The listing builds one solid part. Answer for the finished solid, in the listing's coordinates (mm). A direction names the side the tool comes from. Coordinates: 2 decimals unless noted, no trailing zeros. Loops run counter-clockwise (first coordinate to the right, second up) from the corner with the lowest first, then second, coordinate; pieces in that order, holes last. Notation, with made-up numbers: (59, 9.5) - (64, 9.5) arc R9 ccw to (64, 17.5) - close; hole circle Ø5 at (73, 78). An arc over 180 degrees is marked (long way). Use one line per item in the form item = value. Start each with the question number.
```python
from build123d import *

# Parameters (mm, degrees)
ESQUISSE1_R                  = 13
BASE_EXTRUSION_DEPTH         = 5
ESQUISSE2_R                  = 5
BOSS_EXTRU_1_DEPTH           = 1.1
ESQUISSE3_R                  = 4
BOSS_EXTRU_2_DEPTH           = 16
ESQUISSE4_R                  = 3.5
BOSS_EXTRU_3_DEPTH           = 15
ESQUISSE5_R                  = 2
ENL_V_MAT_EXTRU_1_DEPTH      = 6
R_P_TITION_CIRCULAIRE1_COUNT = 3
ESQUISSE6_W                  = 3.116395494
ESQUISSE6_H                  = 0.94
CHANFREIN1_SIZE              = 0.5
ENL_V_MAT_EXTRU_2_DEPTH      = 10
ESQUISSE9_R                  = 6
ENL_V_MAT_EXTRU_3_DEPTH      = 1


with BuildPart() as part:
    # Esquisse1 → Base-Extrusion (new body)
    with BuildSketch(Plane.XY):
        Circle(ESQUISSE1_R)
    extrude(amount=BASE_EXTRUSION_DEPTH)

    # Esquisse2 → Boss.-Extru.1 (add)
    with BuildSketch(Plane.XY.offset(5)):
        Circle(ESQUISSE2_R)
    extrude(amount=BOSS_EXTRU_1_DEPTH)

    # Esquisse3 → Boss.-Extru.2 (add)
    with BuildSketch(Plane.XY.offset(6.1)):
        Circle(ESQUISSE3_R)
    extrude(amount=BOSS_EXTRU_2_DEPTH)

    # Esquisse4 → Boss.-Extru.3 (add)
    with BuildSketch(Plane.XY.offset(22.1)):
        Circle(ESQUISSE4_R)
    extrude(amount=BOSS_EXTRU_3_DEPTH)

    # Esquisse5 → Enlèv. mat.-Extru.1 (cut, through all)
    with BuildSketch(Plane.XY.offset(5)):
        with Locations((0, 9.75)):
            Circle(ESQUISSE5_R)
    enl_v_mat_extru_1 = extrude(amount=-ENL_V_MAT_EXTRU_1_DEPTH, mode=Mode.SUBTRACT)

    # Répétition circulaire1: Enlèv. mat.-Extru.1 ×3 about axis
    r_p_tition_circulaire1_axis = Axis((0, 0, 0), (0, 0, -1))
    for i in range(1, R_P_TITION_CIRCULAIRE1_COUNT):
        add(enl_v_mat_extru_1.rotate(r_p_tition_circulaire1_axis, i * 360 / R_P_TITION_CIRCULAIRE1_COUNT), mode=Mode.SUBTRACT)

    # Esquisse6 → Enlèvement de matière-Révolution1 (revolve, cut)
    with BuildSketch(Plane(origin=(0, 0, 0), x_dir=(1, 0, 0), z_dir=(0, 1, 0))):
        with Locations((5.058197747, -19.83)):
            Rectangle(ESQUISSE6_W, ESQUISSE6_H)
    revolve(axis=Axis((0, 0, 28.771832847), (0, 0, 1)), mode=Mode.SUBTRACT)

    # Chanfrein1
    chanfrein1_edges = [part.edges().sort_by_distance(p)[0] for p in [
        (-3.5, 0, 37.1),
    ]]
    chamfer(chanfrein1_edges, length=CHANFREIN1_SIZE)

    # Esquisse8 → Enlèv. mat.-Extru.2 (cut)
    with BuildSketch(Plane.XY.offset(37.1)):
        with BuildLine():
            Line((-1.802775638, 3), (1.802775638, 3))
            ThreePointArc((1.802775638, 3), (0, 3.5), (-1.802775638, 3))
        make_face()
    extrude(amount=-ENL_V_MAT_EXTRU_2_DEPTH, mode=Mode.SUBTRACT)

    # Esquisse9 → Enlèv. mat.-Extru.3 (cut)
    with BuildSketch(Plane(origin=(0, 0, 0), x_dir=(-1, 0, 0), z_dir=(0, 0, -1))):
        Circle(ESQUISSE9_R)
    extrude(amount=-ENL_V_MAT_EXTRU_3_DEPTH, mode=Mode.SUBTRACT)


solid = part.part
```
(1) Determine the mould class of faces 4 (the face through (-10.316, -7.91, 2.465)), 5 (the face through (3, -6, 0)), 6 (the face through (-0.26, 11.733, 2.535)) for opening direction Y: +Y half, -Y half, draft (parallel to the pull), parting line (faces both ways), or undercut.
(2) A cutting plane is placed at C-C (z = 12). Determine the outline of the cut face in (x, y).
(3) A cutting plane is placed at D-D (y = -8.5). Determine the outline of the cut face in (x, z).
(4) A cutting plane is placed at A-A (x = -7.75). Determine the outline of the cut face in (y, z), then the cut area to 3 significant figures.
(5) Find the intervals of material crossed by probe 1 along Y at (x, z) = (0, 0.8); probe 2 along Y at (x, z) = (0, 3.15); probe 3 along Z at (x, y) = (-11, -4.75), in increasing order. Write a range as from..to.
(6) Each of these flat-tipped pins is pushed along its axis until it touches: pin 1 Ø4 at (x, z) = (0, 31.5) entering from +Y; pin 2 Ø1.5 at (y, z) = (-2.5, 25) entering from -X; pin 3 Ø1 at (x, y) = (6, 7.5) entering from +Z; pin 4 Ø2.5 at (x, y) = (-8.44, -4.88) entering from +Z. Where does it stop, or does it pass through?
(7) A cutting plane is placed at B-B (y = 9.75). Determine the outline of the cut face in (x, z), then the cut area to 3 significant figures.
(8) For faces 1 (the face through (-0.867, -3.905, 21.187)), 2 (the face through (-2.8, -2.1, 19.8)), 3 (the face through (0, 0, 1)), determine the directions among +Z, -Z, +X, -X, +Y, -Y from which every point of the face is accessible in a straight line to the end or side of a thin tool.
Evaluation:
q1.face_4 = parting line
q1.face_5 = draft
q1.face_6 = undercut
q2.outline = circle Ø8 at (0, 0)
q3.outline = (-9.84, 0) - (9.84, 0) - (9.84, 5) - (-9.84, 5) - close
q4.outline = (-10.44, 0) - (-6.75, 0) - (-6.75, 5) - (-10.44, 5) - close; (-3, 0) - (10.44, 0) - (10.44, 5) - (-3, 5) - close
q4.area = 85.6 mm^2
q5.probe_1 = -13..-6, 6..7.75, 11.75..13
q5.probe_2 = -13..7.75, 11.75..13
q5.probe_3 = 0..5
q6.pin_1 = 3
q6.pin_2 = -3.03
q6.pin_3 = 5
q6.pin_4 = through
q7.outline = (-8.6, 0) - (-2, 0) - (-2, 5) - (-8.6, 5) - close; (2, 0) - (8.6, 0) - (8.6, 5) - (2, 5) - close
q7.area = 66.0 mm^2
q8.face_1 = +Z
q8.face_2 = none
q8.face_3 = -Z
